Source: CAD feature listing. Evaluate the final solid. Frame: model axes, mm. Face numbers are marked on the shaded views. Round coordinates to 2 decimals unless told otherwise and drop trailing zeros. Loops run counter-clockwise (first coordinate to the right, second up) from the corner with the lowest first, then second, coordinate; pieces in that order, holes last. Notation, with made-up numbers: (-9, 25) - (37, 25) arc R21 ccw to (37, 45) - close; hole circle Ø10 at (54.25, 72). An arc over 180 degrees is marked (long way). One line per question, with ' | ' between items. Start each with the question number.
1. Cut plane B-B (x = 67). Return loops of the section in (y, z).
2. Pin query (flat end, axial travel): pin 1 (1.5 mm diameter, centred on y = 8.5, z = 4, fed in from +X); pin 2 (3 mm diameter, centred on x = 95, z = 4, fed in from -Y); pin 3 (1.5 mm diameter, centred on y = 3, z = 4.5, fed in from -X). Return the tip coordinate at first contact, or that it passes through.
3. Mould query, pull axis X, two halves, no side actions, for the marked faces 1 and 2. Classes: pulls with the +X half, pulls with the -X half, needs draft (parallel to the pull), parting line crosses it, or undercut.
4. Ray query, line 1 (X direction, y = 5.75, z = 0.75); line 2 (X direction, y = 6.5, z = 3.5) (3 decimals); line 3 (Y direction, x = 102, z = 2.75). Return the intervals inside material, ascending.
5. Cut plane A-A (z = 4). Return loops of the section in (x, y), then the cut area to 3 significant figures.
6. Cut plane C-C (y = 11). Return loops of the section in (x, z), then the cut area to 3 significant figures.
Solid Edge part; units mm, degrees
sketch "Sketch1" plane through (0, 0, 0) normal (0, 0, -1) x (-1, 0, 0)
  circle A0 centre (-7.5774, 7.5955) radius 2.032
  circle A1 centre (-42.5636, 7.5955) radius 2.032
  circle A2 centre (-122.4658, 7.5955) radius 2.032
  line L0 (-121.5515, 12.6669) -> (-42.6073, 15.0526)
  line L1 (-42.6073, 15.0526) -> (-7.5579, 14.9599)
  arc A3 (-7.5579, 14.9599) -> (-13.1588, 2.7909) centre (-7.5774, 7.5955) cw
  arc A4 (-17.0309, 4.6448) -> (-13.1588, 2.7909) centre (-18.673, -3.7556) cw
  arc A5 (-33.2754, 4.6448) -> (-17.0309, 4.6448) centre (-25.1531, -63.7101) cw
  arc A6 (-42.7786, 0.1413) -> (-33.2754, 4.6448) centre (-44.3624, 15.762) ccw
  line L2 (-122.6144, 2.4444) -> (-42.7786, 0.1413)
  arc A7 (-121.5515, 12.6669) -> (-122.6144, 2.4444) centre (-122.4658, 7.5955) ccw
extrude "Protrusion1" add sketch "Sketch1" against normal blind 7.9502
properties part number "AC_1.07"
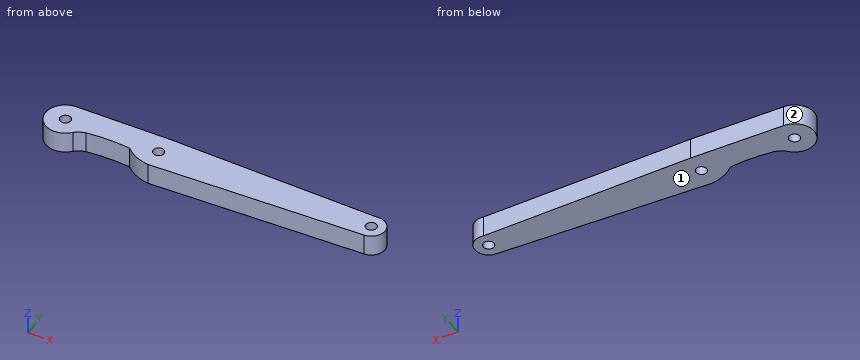
Answers follow:
1) outline: (0.84, 0) - (14.32, 0) - (14.32, 7.95) - (0.84, 7.95) - close
2) pin 1: stops at x = 127.62 | pin 2: stops at y = 1.6 | pin 3: stops at x = 1.3
3) face 1: needs draft | face 2: undercut
4) line 1: x = 0.45 to 6.73, 8.43 to 41.71, 43.41 to 121.62, 123.32 to 127.28 | line 2: x = 0.295 to 5.866, 9.289 to 40.852, 44.275 to 120.754, 124.177 to 127.501 | line 3: y = 1.85 to 13.26
5) outline: (7.56, 14.96) arc R7.36 ccw (long way) to (13.16, 2.79) arc R8.56 cw to (17.03, 4.64) arc R68.84 cw to (33.28, 4.64) arc R15.7 ccw to (42.78, 0.14) - (122.61, 2.44) arc R5.15 ccw (long way) to (121.55, 12.67) - (42.61, 15.05) - close; hole circle Ø4.06 at (7.58, 7.6); hole circle Ø4.06 at (42.56, 7.6); hole circle Ø4.06 at (122.47, 7.6) | area: 1,500 mm2
6) outline: (1.05, 0) - (126.33, 0) - (126.33, 7.95) - (1.05, 7.95) - close | area: 996 mm2
